from build123d import *

# Parameters (mm, degrees)
SKETCH_1_R               = 5
EXTRUDE_1_DEPTH          = 21
SKETCH_2_R               = 5.5
EXTRUDE_2_DEPTH          = 1.2
SKETCH_3_R               = 6
EXTRUDE_3_DEPTH          = 38
SKETCH_4_R               = 5.5
EXTRUDE_4_DEPTH          = 1.2
SKETCH_5_R               = 6
EXTRUDE_5_DEPTH          = 24
SKETCH_6_R               = 3.25
EXTRUDE_6_DEPTH          = 3
SKETCH_7_R               = 4
EXTRUDE_7_DEPTH          = 14
SKETCH_9_OUTSIDE_W       = 34.76
SKETCH_9_OUTSIDE_H       = 34.76
CUT_EXTRUDE_1_DEPTH      = 19
EXTRUDE_8_DEPTH          = 21
PATTERN_CIRCULAR_1_COUNT = 8


# Read off the part's stored shape, not the designer's step: M8 机械螺纹 螺柱1
with BuildPart() as part:
    # 草图1 → 凸台-拉伸1 (new body)
    with BuildSketch(Plane.XY):
        with Locations(Location((0, 0, 0), (0, 0, 180))):
            Circle(SKETCH_1_R)
    extrude(amount=EXTRUDE_1_DEPTH)

    # 草图2 → 凸台-拉伸2 (add)
    with BuildSketch(Plane.XY.offset(21)):
        Circle(SKETCH_2_R)
    extrude(amount=EXTRUDE_2_DEPTH)

    # 草图3 → 凸台-拉伸3 (add)
    with BuildSketch(Plane.XY.offset(22.2)):
        Circle(SKETCH_3_R)
    extrude(amount=EXTRUDE_3_DEPTH)

    # 草图4 → 凸台-拉伸4 (add)
    with BuildSketch(Plane.XY.offset(60.2)):
        Circle(SKETCH_4_R)
    extrude(amount=EXTRUDE_4_DEPTH)

    # 草图5 → 凸台-拉伸5 (add)
    with BuildSketch(Plane.XY.offset(61.4)):
        Circle(SKETCH_5_R)
    extrude(amount=EXTRUDE_5_DEPTH)

    # 草图6 → 凸台-拉伸6 (add)
    with BuildSketch(Plane.XY.offset(85.4)):
        Circle(SKETCH_6_R)
    extrude(amount=EXTRUDE_6_DEPTH)

    # 草图7 → 凸台-拉伸7 (add)
    with BuildSketch(Plane.XY.offset(88.4)):
        Circle(SKETCH_7_R)
    extrude(amount=EXTRUDE_7_DEPTH)

    # M8 机械螺纹 螺柱1 outline → M8 机械螺纹 螺柱1 (revolve, cut)
    with BuildSketch(Plane.XZ):
        Polygon((4, 102.4), (3.3235, 102.4), (4, 101.7235), align=None)
    revolve(axis=Axis((0, 0, 0), (0, 0, 1)), mode=Mode.SUBTRACT)

    # 草图9 outside → 切除-拉伸1 (cut)
    with BuildSketch(Plane.XY.offset(85.4)):
        Rectangle(SKETCH_9_OUTSIDE_W, SKETCH_9_OUTSIDE_H)
        Polygon((0, -6.363961031), (6.363961031, 0), (0, 6.363961031), (-6.363961031, 0), align=None, mode=Mode.SUBTRACT)
    extrude(amount=-CUT_EXTRUDE_1_DEPTH, mode=Mode.SUBTRACT)

    # 草图10 → 凸台-拉伸8 (add)
    with BuildSketch(Plane(origin=(0, 0, 0), x_dir=(-1, 0, 0), z_dir=(0, 0, -1))):
        with BuildLine():
            ThreePointArc((1, 5.916079783), (0, 6), (-1, 5.916079783))
            Line((-1, 5.916079783), (-1, 4.898979486))
            ThreePointArc((-1, 4.898979486), (0, 5), (1, 4.898979486))
            Line((1, 4.898979486), (1, 5.916079783))
        make_face()
    extrude_8 = extrude(amount=-EXTRUDE_8_DEPTH)

    # 阵列(圆周)1: 凸台-拉伸8 ×8 about axis
    pattern_circular_1_axis = Axis((0, 0, 0), (0, 0, 1))
    for i in range(1, PATTERN_CIRCULAR_1_COUNT):
        add(extrude_8.rotate(pattern_circular_1_axis, i * 360 / PATTERN_CIRCULAR_1_COUNT))


solid = part.part
Input: part model. Units: mm. Frame: model coordinates. A direction names the side the tool comes from. Give positions to 0.01 mm unless a question says otherwise; leave off trailing zeros. Write each loop counter-clockwise with the first axis right and the second up, starting at its lowest first coordinate (ties: lowest second). Pieces come first, ordered by that corner, then holes. Notation, with made-up numbers: M 17.25,-17.75 L 47.25,-17.75 A23 ccw 47.25,1.25 Z; hole C 19.25,79 d10. An arc over 180 degrees is marked long. Use one line per item in the form item = value.
1. Ray query, L1, parallel to X at y = 4.5, z = 9.5; L2, parallel to Z at x = 4.25, y = 2.75; L3, parallel to Z at x = 4.5, y = 1. Return the intervals inside material, ascending.
Outcome:
L1 = -3.97 to -3.09, -2.18 to 2.18, 3.09 to 3.97
L2 = 21 to 66.4
L3 = 0 to 85.4
2. Reachability of faces 1 (the face through (-1.926, -4.614, 10.353)), 2 (the face through (3, -5, 22.2)), 3 (the face through (-3.143, 3.221, 76.033)), 4 (the face through (-3.221, -3.143, 76.033)) from +Z, -Z, +X, -X, +Y, -Y: full face, straight path, thin tool, end or side. Return the list, or none.
Outcome:
face_1 = -Z, -Y
face_2 = none
face_3 = +Z, -X, +Y
face_4 = +Z, -X, -Y
3. First-contact query: P1, Ø2, axis at x = 2.5, y = 4, coming from the -Z side; P2, Ø6, axis at y = -4.5, z = 22, coming from the +X side; P3, Ø2, axis at y = 4.5, z = 65, coming from the +X side; P4, Ø0.8, axis at x = 5.5, z = 13.5, coming from the -Y side. Flat tips, straight axial feed; report the tip coordinate or a pass-through.
Outcome:
P1 = 0
P2 = 5.81
P3 = 4.87
P4 = -1
4. Mould query, pull axis Z, two halves, no side actions, for faces 5 (the face through (-4.614, 1.926, 10.353)), 6 (the face through (0, 0, 0)), 7 (the face through (-1.19, -5.37, 60.79)). Classes: released by +Z, released by -Z, zero draft, split by the parting line, or undercut.
Outcome:
face_5 = zero draft
face_6 = released by -Z
face_7 = undercut
5. Cut plane B-B on z = 29.5. Return loops of the section in (x, y), and give its area (3 significant figures).
Outcome:
outline = C 0,0 d12
area = 113 mm²
